```python
from build123d import *

# Parameters (mm, degrees)
SKETCH_1_R      = 2.6
EXTRUDE_1_DEPTH = 38.75
FILLET_1_R      = 1.5
FILLET_2_R      = 0.3


with BuildPart() as part:
    # 草图1 → 凸台-拉伸1 (new, symmetric)
    with BuildSketch(Plane.XY):
        Polygon((-13.9, 0), (-13.9, 2.839339828), (-16.560660172, 5.5), (-18.2, 5.5), (-18.2, 3.1), (-19.4, 3.1), (-19.4, 3.6), (-20, 3.6), (-20, 10), (-13.6, 10), (-13.6, 9.4), (-13.1, 9.4), (-13.1, 8.2), (-15.5, 8.2), (-15.5, 6.560660172), (-12.839339828, 3.9), (-7.160660172, 3.9), (-4.5, 6.560660172), (-4.5, 8.2), (-6.9, 8.2), (-6.9, 9.4), (-6.4, 9.4), (-6.4, 10), (6.4, 10), (6.4, 9.4), (6.9, 9.4), (6.9, 8.2), (4.5, 8.2), (4.5, 6.560660172), (7.160660172, 3.9), (12.839339828, 3.9), (15.5, 6.560660172), (15.5, 8.2), (13.1, 8.2), (13.1, 9.4), (13.6, 9.4), (13.6, 10), (20, 10), (20, 3.6), (19.4, 3.6), (19.4, 3.1), (18.2, 3.1), (18.2, 5.5), (16.560660172, 5.5), (13.9, 2.839339828), (13.9, 0), (13.9, -2.839339828), (16.560660172, -5.5), (18.2, -5.5), (18.2, -3.1), (19.4, -3.1), (19.4, -3.6), (20, -3.6), (20, -10), (13.6, -10), (13.6, -9.4), (13.1, -9.4), (13.1, -8.2), (15.5, -8.2), (15.5, -6.560660172), (12.839339828, -3.9), (7.160660172, -3.9), (4.5, -6.560660172), (4.5, -8.2), (6.9, -8.2), (6.9, -9.4), (6.4, -9.4), (6.4, -10), (-6.4, -10), (-6.4, -9.4), (-6.9, -9.4), (-6.9, -8.2), (-4.5, -8.2), (-4.5, -6.560660172), (-7.160660172, -3.9), (-12.839339828, -3.9), (-15.5, -6.560660172), (-15.5, -8.2), (-13.1, -8.2), (-13.1, -9.4), (-13.6, -9.4), (-13.6, -10), (-20, -10), (-20, -3.6), (-19.4, -3.6), (-19.4, -3.1), (-18.2, -3.1), (-18.2, -5.5), (-16.560660172, -5.5), (-13.9, -2.839339828), align=None)
        with Locations((-10, 0)):
            Circle(SKETCH_1_R, mode=Mode.SUBTRACT)
        with Locations(Location((10, 0, 0), (0, 0, 180))):
            Circle(SKETCH_1_R, mode=Mode.SUBTRACT)
        Polygon((-6.1, -2.839339828), (-6.1, 2.839339828), (-2.7, 6.239339828), (-2.7, 8.2), (2.7, 8.2), (2.7, 6.239339828), (6.1, 2.839339828), (6.1, -2.839339828), (2.7, -6.239339828), (2.7, -8.2), (-2.7, -8.2), (-2.7, -6.239339828), align=None, mode=Mode.SUBTRACT)
    extrude(amount=EXTRUDE_1_DEPTH, both=True)

    # 圆角1
    fillet_1_edges = [part.edges().sort_by_distance(p)[0] for p in [
        (-20, 10, 0),
        (20, 10, 0),
        (20, -10, 0),
        (-20, -10, 0),
    ]]
    fillet(fillet_1_edges, radius=FILLET_1_R)

    # 圆角2
    fillet_2_edges = [part.edges().sort_by_distance(p)[0] for p in [
        (-20, 3.6, 0),
        (-13.6, 10, 0),
        (-6.4, 10, 0),
        (6.4, 10, 0),
        (13.6, 10, 0),
        (20, 3.6, 0),
        (20, -3.6, 0),
        (13.6, -10, 0),
        (6.4, -10, 0),
        (-6.4, -10, 0),
        (-13.6, -10, 0),
        (-20, -3.6, 0),
    ]]
    fillet(fillet_2_edges, radius=FILLET_2_R)


solid = part.part
```
Here's how the part is built. I have some questions about the finished solid (model axes, mm). A direction names the side the tool comes from. Round coordinates to 2 decimals unless told otherwise and drop trailing zeros. Write each loop counter-clockwise with the first axis right and the second up, starting at its lowest first coordinate (ties: lowest second). Pieces come first, ordered by that corner, then holes.
Q1. Will these pins go through, and if not, where does the flat tip stop? P1, Ø8, axis at x = -10, z = 13, coming from the +Y side; P2, Ø0.6, axis at y = 3.5, z = -16, coming from the -X side; P3, Ø4, axis at x = -10, z = -4.5, coming from the +Y side; P4, Ø1.5, axis at y = 0, z = 17, coming from the +X side.
Q2. If we section it at A-A on y = 0: Write out the boundary of the cut face in (x, z), plus the area to 3 significant figures.
Q3. If we section it at B-B on x = 10: Write out the boundary of the cut face in (y, z), plus the area to 4 significant figures.
Q4. If we mould it in two halves opening along X, with no side actions, what happens to faces 4 (the cylindrical face through (19.57, -9.55, 0.54)), 5 (the cylindrical face through (-19.57, 9.55, -0.54)), 6 (the flat face through (18.2, 4, 1))? For each: +X half, -X half, draft (parallel to the pull), parting line (faces both ways), or undercut.
Q5. Please list where these lines run through material, in increasing order: probe 1 along X at (y, z) = (7, 0); probe 2 along X at (y, z) = (0.75, -20.5); probe 3 along Y at (x, z) = (-10, 22).
Q6. Which directions (+Z, -Z, +X, -X, +Y, -Y) give clear straight access to the entire face, cutting with the end or side of a thin tool? Please do faces 1 (the flat face through (-10, 3.9, 1)), 2 (the flat face through (4.38, 4.56, 0.54)), 3 (the flat face through (-20, -6, 1)).
Q7. If we section it at C-C on z = -26: Give the number of separate pieces and of enclosed holes in the cut face, plus the area to 3 significant figures.
Answer below:
1. P1: stops at y = 10
1. P2: stops at x = -19.98
1. P3: stops at y = 3.9
1. P4: stops at x = 13.9
2. outline: (-13.9, -38.75) - (-12.6, -38.75) - (-12.6, 38.75) - (-13.9, 38.75) - close; (-7.4, -38.75) - (-6.1, -38.75) - (-6.1, 38.75) - (-7.4, 38.75) - close; (6.1, -38.75) - (7.4, -38.75) - (7.4, 38.75) - (6.1, 38.75) - close; (12.6, -38.75) - (13.9, -38.75) - (13.9, 38.75) - (12.6, 38.75) - close
2. area: 403 mm2
3. outline: (-3.9, -38.75) - (-2.6, -38.75) - (-2.6, 38.75) - (-3.9, 38.75) - close; (2.6, -38.75) - (3.9, -38.75) - (3.9, 38.75) - (2.6, 38.75) - close
3. area: 201.5 mm2
4. face 4: +X half
4. face 5: -X half
4. face 6: undercut
5. probe 1: x = -20 to -15.5, -4.5 to -2.7, 2.7 to 4.5, 15.5 to 20
5. probe 2: x = -13.9 to -12.49, -7.51 to -6.1, 6.1 to 7.51, 12.49 to 13.9
5. probe 3: y = -3.9 to -2.6, 2.6 to 3.9
6. face 1: +Z, -Z, +Y
6. face 2: +Z, -Z
6. face 3: +Z, -Z, -X, +Y, -Y
7. separate pieces: 1
7. enclosed holes: 3
7. area: 293 mm2
